from build123d import *

# Parameters (mm, degrees)
SKETCH1_W           = 12
SKETCH1_H           = 11
BOSS_EXTRUDE1_DEPTH = 20
SKETCH2_R           = 1.5
BOSS_EXTRUDE2_DEPTH = 19
SKETCH3_R           = 3.5
BOSS_EXTRUDE3_DEPTH = 1
SKETCH4_R           = 2
BOSS_EXTRUDE4_DEPTH = 1
SKETCH5_R           = 1
CUT_EXTRUDE1_DEPTH  = 12


with BuildPart() as part:
    # Sketch1 → Boss-Extrude1 (new body)
    with BuildSketch(Plane(origin=(0, 0, 0), x_dir=(1, 0, 0), z_dir=(0, 1, 0))):
        with Locations((6, 5.5)):
            Rectangle(SKETCH1_W, SKETCH1_H)
    extrude(amount=BOSS_EXTRUDE1_DEPTH)

    # Sketch2 → Boss-Extrude2 (add)
    with BuildSketch(Plane(origin=(0, 20, 0), x_dir=(1, 0, 0), z_dir=(0, 1, 0))):
        with Locations(Location((6, 5.5, 0), (0, 0, 270))):
            Circle(SKETCH2_R)
    extrude(amount=BOSS_EXTRUDE2_DEPTH)

    # Sketch3 → Boss-Extrude3 (add)
    with BuildSketch(Plane(origin=(0, 27, 0), x_dir=(1, 0, 0), z_dir=(0, 1, 0))):
        with Locations(Location((6, 5.5, 0), (0, 0, 270))):
            Circle(SKETCH3_R)
    extrude(amount=BOSS_EXTRUDE3_DEPTH)

    # Sketch4 → Boss-Extrude4 (add)
    with BuildSketch(Plane(origin=(0, 28, 0), x_dir=(1, 0, 0), z_dir=(0, 1, 0))):
        with Locations(Location((6, 5.5, 0), (0, 0, 270))):
            Circle(SKETCH4_R)
    extrude(amount=BOSS_EXTRUDE4_DEPTH)

    # Sketch5 → Cut-Extrude1 (cut)
    with BuildSketch(Plane(origin=(12, 0, 0), x_dir=(0, 0, -1), z_dir=(1, 0, 0))):
        with Locations((2.25, 4.5)):
            Circle(SKETCH5_R)
        with Locations((8.75, 14.5)):
            Circle(SKETCH5_R)
    extrude(amount=-CUT_EXTRUDE1_DEPTH, mode=Mode.SUBTRACT)


solid = part.part
Input: part model. Units: mm. Frame: model coordinates. A direction names the side the tool comes from. Round coordinates to 2 decimals unless told otherwise and drop trailing zeros. Write each loop counter-clockwise with the first axis right and the second up, starting at its lowest first coordinate (ties: lowest second). Pieces come first, ordered by that corner, then holes.
1) Cut plane D-D (z = -5.5). Return the cut outline in (x, y), then the cut area to 3 significant figures.
2) Cut plane B-B (x = 6). Return the cut outline in (y, z).
3) Contact query for flat-ended pins moving along their axis: P1, Ø1.8, axis at y = 14.5, z = -8.75, coming from the -X side; P2, Ø2, axis at x = 3.5, z = -7.5, coming from the +Y side. Output: stop coordinate, or through.
4) Reachability of faces 1 (the flat face through (4, 27, -6)), 2 (the cylindrical face through (6.084, 5.176, -1.513)), 3 (the cylindrical face through (6, 34, -7)) from +Z, -Z, +X, -X, +Y, -Y: full face, straight path, thin tool, end or side. Return the list, or none.
5) Cut plane C-C (z = -8.5). Return the cut outline in (x, y), then the cut area to 3 significant figures.
6) Ray query, L1, parallel to Y at x = 5, z = -2.25; L2, parallel to Y at x = 3, z = -2.25; L3, parallel to Y at x = 2.5, z = -6.25. Return the intervals inside material, ascending.
7) Draft query along Y for faces 4 (the flat face through (7, 29, -7)), 5 (the flat face through (5, 20, -7)), 6 (the flat face through (0, 10, -5)). Return one class per face: pulls with the +Y half, pulls with the -Y half, needs draft (parallel to the pull), parting line crosses it, or undercut.
8) Cut plane A-A (y = 4.5). Return the cut outline in (x, z).
Geometry says:
1. outline: (0, 0) - (12, 0) - (12, 20) - (7.5, 20) - (7.5, 27) - (9.5, 27) - (9.5, 28) - (8, 28) - (8, 29) - (7.5, 29) - (7.5, 39) - (4.5, 39) - (4.5, 29) - (4, 29) - (4, 28) - (2.5, 28) - (2.5, 27) - (4.5, 27) - (4.5, 20) - (0, 20) - close
1. area: 302 mm2
2. outline: (0, -11) - (20, -11) - (20, -7) - (27, -7) - (27, -9) - (28, -9) - (28, -7.5) - (29, -7.5) - (29, -7) - (39, -7) - (39, -4) - (29, -4) - (29, -3.5) - (28, -3.5) - (28, -2) - (27, -2) - (27, -4) - (20, -4) - (20, 0) - (0, 0) - close; hole circle Ø2 at (4.5, -2.25); hole circle Ø2 at (14.5, -8.75)
3. P1: passes through
3. P2: stops at y = 28
4. face 1: none
4. face 2: +X, -X
4. face 3: +Y
5. outline: (0, 0) - (12, 0) - (12, 13.53) - (0, 13.53) - close; (0, 15.47) - (12, 15.47) - (12, 20) - (0, 20) - close; (4.2, 27) - (7.8, 27) - (7.8, 28) - (4.2, 28) - close
5. area: 220 mm2
6. L1: y = 0 to 3.5, 5.5 to 20, 27 to 28
6. L2: y = 0 to 3.5, 5.5 to 20
6. L3: y = 0 to 20
7. face 4: pulls with the +Y half
7. face 5: undercut
7. face 6: needs draft
8. outline: (0, -11) - (12, -11) - (12, -3.25) - (0, -3.25) - close; (0, -1.25) - (12, -1.25) - (12, 0) - (0, 0) - close
